Source: CAD feature listing. Evaluate the final solid. Frame: model axes, mm. Round coordinates to 2 decimals unless told otherwise and drop trailing zeros. Write each loop counter-clockwise with the first axis right and the second up, starting at its lowest first coordinate (ties: lowest second). Pieces come first, ordered by that corner, then holes. Notation, with made-up numbers: M 9.5,20 L 65.5,20 A24 cw 65.5,31 Z; hole C -15,26.5 d3. An arc over 180 degrees is marked long. Use a Markdown table: item, result.
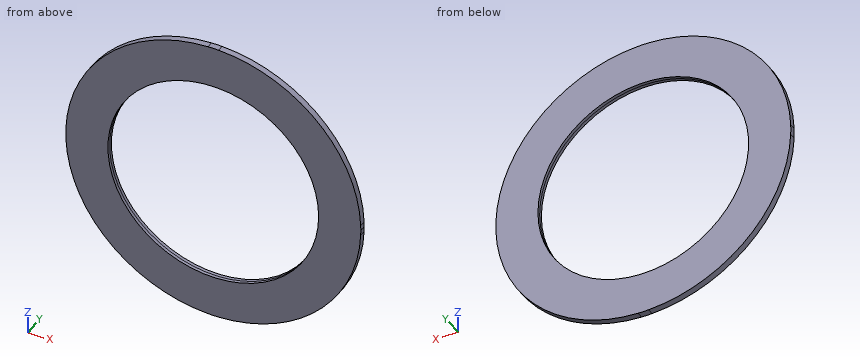
```python
from build123d import *

# Parameters (mm, degrees)
F_98MM_6ID_CENTERING_RING_SKETCH_7_R = 63.5
CENTERING_RING_EXTRUDE_DEPTH         = 1.905
CENTERING_RING_EXTRUDE_DEPTH_BACK    = 1.905


with BuildPart() as part:
    # 98mm - 6ID centering ring sketch_7 → Centering Ring Extrude (new body, two sides)
    with BuildSketch(Plane(origin=(0, 0, 0), x_dir=(1, 0, 0), z_dir=(0, 1, 0))) as centering_ring_extrude_sk:
        with BuildLine():
            Line((66.599361859, 3.175), (88.843285481, 3.175))
            ThreePointArc((88.843285481, 3.175), (62.861792847, 62.861792847), (3.175, 88.843285481))
            Line((3.175, 88.843285481), (3.175, 66.599361859))
            ThreePointArc((3.175, 66.599361859), (0, 66.675), (-3.175, 66.599361859))
            Line((-3.175, 66.599361859), (-3.175, 88.843285481))
            ThreePointArc((-3.175, 88.843285481), (-62.861792847, 62.861792847), (-88.843285481, 3.175))
            Line((-88.843285481, 3.175), (-66.599361859, 3.175))
            ThreePointArc((-66.599361859, 3.175), (-66.675, 0), (-66.599361859, -3.175))
            Line((-66.599361859, -3.175), (-88.843285481, -3.175))
            ThreePointArc((-88.843285481, -3.175), (-62.861792847, -62.861792847), (-3.175, -88.843285481))
            Line((-3.175, -88.843285481), (-3.175, -66.599361859))
            ThreePointArc((-3.175, -66.599361859), (0, -66.675), (3.175, -66.599361859))
            Line((3.175, -66.599361859), (3.175, -88.843285481))
            ThreePointArc((3.175, -88.843285481), (62.861792847, -62.861792847), (88.843285481, -3.175))
            Line((88.843285481, -3.175), (66.599361859, -3.175))
            ThreePointArc((66.599361859, -3.175), (66.675, 0), (66.599361859, 3.175))
        make_face()
        Circle(F_98MM_6ID_CENTERING_RING_SKETCH_7_R, mode=Mode.SUBTRACT)
        with BuildLine():
            ThreePointArc((88.9, 0), (88.885820239, 1.58775325), (88.843285481, 3.175))
            Line((88.843285481, 3.175), (66.599361859, 3.175))
            ThreePointArc((66.599361859, 3.175), (66.675, 0), (66.599361859, -3.175))
            Line((66.599361859, -3.175), (88.843285481, -3.175))
            ThreePointArc((88.843285481, -3.175), (88.885820239, -1.58775325), (88.9, 0))
        make_face()
        with BuildLine():
            Line((3.175, 66.599361859), (3.175, 88.843285481))
            ThreePointArc((3.175, 88.843285481), (0, 88.9), (-3.175, 88.843285481))
            Line((-3.175, 88.843285481), (-3.175, 66.599361859))
            ThreePointArc((-3.175, 66.599361859), (0, 66.675), (3.175, 66.599361859))
        make_face()
        with BuildLine():
            Line((-66.599361859, 3.175), (-88.843285481, 3.175))
            ThreePointArc((-88.843285481, 3.175), (-88.9, 0), (-88.843285481, -3.175))
            Line((-88.843285481, -3.175), (-66.599361859, -3.175))
            ThreePointArc((-66.599361859, -3.175), (-66.675, 0), (-66.599361859, 3.175))
        make_face()
        with BuildLine():
            ThreePointArc((-3.175, -88.843285481), (0, -88.9), (3.175, -88.843285481))
            Line((3.175, -88.843285481), (3.175, -66.599361859))
            ThreePointArc((3.175, -66.599361859), (0, -66.675), (-3.175, -66.599361859))
            Line((-3.175, -66.599361859), (-3.175, -88.843285481))
        make_face()
    extrude(amount=CENTERING_RING_EXTRUDE_DEPTH)
    extrude(centering_ring_extrude_sk.sketch, amount=-CENTERING_RING_EXTRUDE_DEPTH_BACK)


solid = part.part
```
Q1. Section D-D on x = 77. Return loops of the section in (y, z) (3 decimals), plus the area to 3 significant figures.
Results are:
| item | result |
|---|---|
| outline | M -1.905,-44.432 L 1.905,-44.432 L 1.905,44.432 L -1.905,44.432 Z |
| area | 339 mm^2 |
Q2. First-contact query: pin 1 Ø2 at (x, y) = (-31.5, 1) entering from +Z; pin 2 Ø2 at (y, z) = (1, 16.5) entering from +X. Flat tips, straight axial feed; report the tip coordinate or a pass-through.
Results are:
| item | result |
|---|---|
| pin 1 | z = 83.5 |
| pin 2 | x = 87.54 |
Q3. Line query: L1, parallel to Z at x = 0, y = -0.8; L2, parallel to Z at x = -10.5, y = 1; L3, parallel to X at y = -1.55, z = -24. Output: solid intervals per line, ascending.
Results are:
| item | result |
|---|---|
| L1 | -88.9 to -63.5, 63.5 to 88.9 |
| L2 | -88.28 to -62.63, 62.63 to 88.28 |
| L3 | -85.6 to -58.79, 58.79 to 85.6 |
Q4. Section C-C on z = 21.5. Return loops of the section in (x, y) (3 decimals).
Results are:
| item | result |
|---|---|
| outline | M -86.261,-1.905 L -59.749,-1.905 L -59.749,1.905 L -86.261,1.905 Z; M 59.749,-1.905 L 86.261,-1.905 L 86.261,1.905 L 59.749,1.905 Z |
Q5. Section B-B on y = 1.2. Return loops of the section in (x, z) (3 decimals).
Results are:
| item | result |
|---|---|
| outline | M 88.843,-3.175 A88.9 ccw 88.843,3.175 A88.9 ccw long Z; hole C 0,0 d127 |
Q6. Section A-A on x = 0. Return loops of the section in (y, z) (3 decimals), plus the area to 3 significant figures.
Results are:
| item | result |
|---|---|
| outline | M -1.905,-88.9 L 1.905,-88.9 L 1.905,-63.5 L -1.905,-63.5 Z; M -1.905,63.5 L 1.905,63.5 L 1.905,88.9 L -1.905,88.9 Z |
| area | 194 mm^2 |
